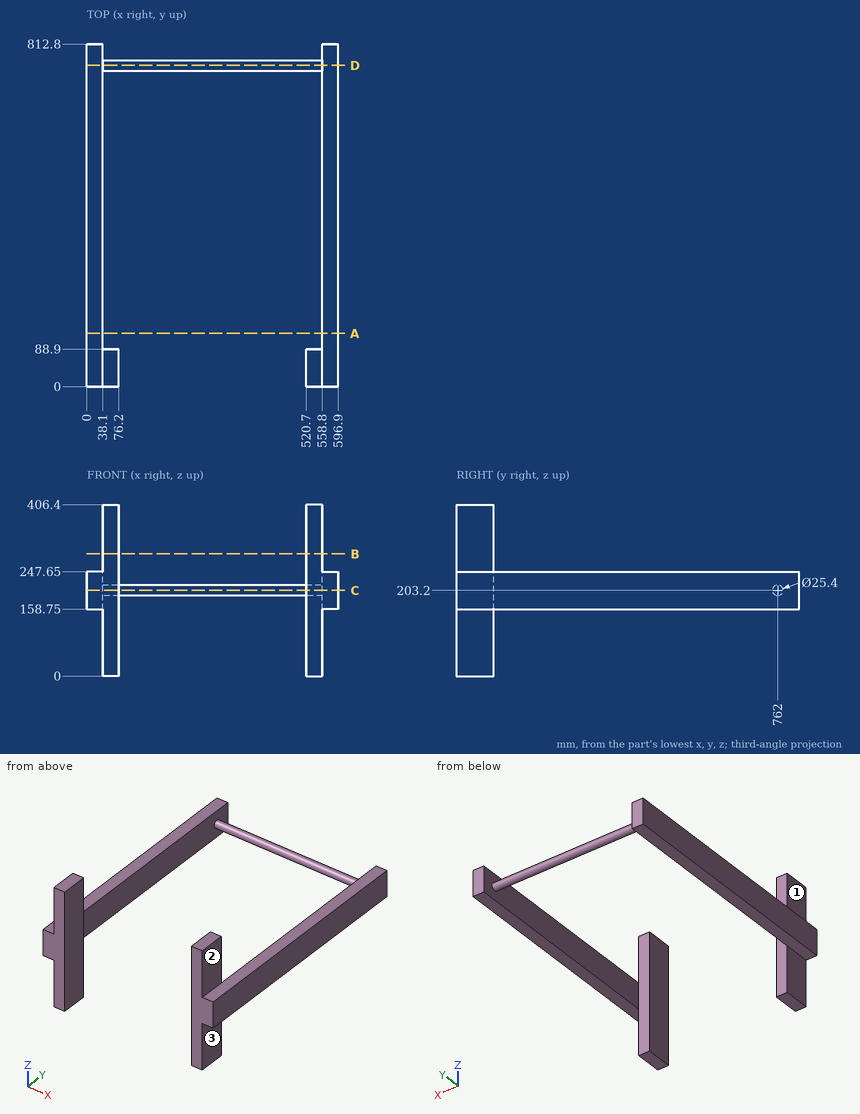
Answer from the drawing. Dimensions are ordinates in mm from the lowest x, y and z of the part. A direction names the side the tool comes from. Give positions to 0.01 mm unless a question says otherwise; leave off trailing zeros. Write each loop counter-clockwise with the first axis right and the second up, starting at its lowest first coordinate (ties: lowest second). Pieces come first, ordered by that corner, then holes. Notation, with made-up numbers: (-1.75, 62.5) -> (32.25, 62.5) arc R25 ccw to (32.25, 85.5) -> close; hole circle Ø9 at (-10, 83). An arc over 180 degrees is marked (long way). Use a Markdown table: item, result.
(1) For the marked faces 1, 2 and 3, determine the directions among +Z, -Z, +X, -X, +Y, -Y from which every point of the face is accessible in a straight line to the end or side of a thin tool.
Return value:
| item | result |
|---|---|
| face 1 | +Z, -X, +Y, -Y |
| face 2 | +Z, +X, +Y, -Y |
| face 3 | -Z, +X, +Y, -Y |
(2) Flat-ended cylindrical pins translate along their axes: P1, Ø11.5, axis at x = 61.5, z = 270, coming from the +Y side; P2, Ø19, axis at x = 574.5, y = 590.5, coming from the +Z side. Find the tip coordinate at first contact, or state that the pin passes through.
Return value:
| item | result |
|---|---|
| P1 | y = 88.9 |
| P2 | z = 247.65 |
(3) Section C-C, the plane z = 203.2 is taken. Determine the outline of the cut face in (x, y), then the cut area to 3 significant figures.
Return value:
| item | result |
|---|---|
| outline | (0, 0) -> (76.2, 0) -> (76.2, 88.9) -> (38.1, 88.9) -> (38.1, 749.3) -> (558.8, 749.3) -> (558.8, 88.9) -> (520.7, 88.9) -> (520.7, 0) -> (596.9, 0) -> (596.9, 812.8) -> (558.8, 812.8) -> (558.8, 774.7) -> (38.1, 774.7) -> (38.1, 812.8) -> (0, 812.8) -> close |
| area | 81,900 mm2 |
(4) Find the intervals of material crossed by probe 1 along X at (y, z) = (432.5, 227); probe 2 along Y at (x, z) = (39, 76); probe 3 along X at (y, z) = (57, 129.5), in increasing order. Write a range as from..to.
Return value:
| item | result |
|---|---|
| probe 1 | 0..38.1, 558.8..596.9 |
| probe 2 | 0..88.9 |
| probe 3 | 38.1..76.2, 520.7..558.8 |
(5) Section A-A, the plane y = 126.5 is taken. Determine the outline of the cut face in (x, z).
Return value:
| item | result |
|---|---|
| outline | (0, 158.75) -> (38.1, 158.75) -> (38.1, 247.65) -> (0, 247.65) -> close; (558.8, 158.75) -> (596.9, 158.75) -> (596.9, 247.65) -> (558.8, 247.65) -> close |
(6) Section D-D, the plane y = 762 is taken. Determine the outline of the cut face in (x, z).
Return value:
| item | result |
|---|---|
| outline | (0, 158.75) -> (38.1, 158.75) -> (38.1, 190.5) -> (558.8, 190.5) -> (558.8, 158.75) -> (596.9, 158.75) -> (596.9, 247.65) -> (558.8, 247.65) -> (558.8, 215.9) -> (38.1, 215.9) -> (38.1, 247.65) -> (0, 247.65) -> close |
(7) Section B-B, the plane z = 289.5 is taken. Determine the outline of the cut face in (x, y), then the cut area to 3 significant figures.
Return value:
| item | result |
|---|---|
| outline | (38.1, 0) -> (76.2, 0) -> (76.2, 88.9) -> (38.1, 88.9) -> close; (520.7, 0) -> (558.8, 0) -> (558.8, 88.9) -> (520.7, 88.9) -> close |
| area | 6,770 mm2 |
